Read the model definition and answer for the solid it produces. Units are mm, in the model's axes. Face numbers are marked on the shaded views. A direction names the side the tool comes from. Give positions to 0.01 mm unless a question says otherwise; leave off trailing zeros. Order: outer loops, then holes, each group sorted by start corner. A loop starts at its lowest first (then second) coordinate and runs counter-clockwise, first axis right, second up. Notation, with made-up numbers: (80.25, 30) - (137.25, 30) arc R30 ccw to (137.25, 69) - close; hole circle Ø3 at (-38, -8.75). An arc over 180 degrees is marked (long way). Write each question's results on one line, items separated by ' | '.
from build123d import *

# Parameters (mm, degrees)
F1_DEPTH = 2
F2_DEPTH = 8
F3_DEPTH = 7.25


with BuildPart() as f1:
    # F0 (on Top) → F1 (new body)
    with BuildSketch(Plane.XY):
        with BuildLine():
            Line((4.85, 7.2), (-4.85, 7.2))
            ThreePointArc((-4.85, 7.2), (-6.511701, 6.511701), (-7.2, 4.85))
            Line((-7.2, 4.85), (-7.2, -4.85))
            ThreePointArc((-7.2, -4.85), (-6.511701, -6.511701), (-4.85, -7.2))
            Line((-4.85, -7.2), (4.85, -7.2))
            ThreePointArc((4.85, -7.2), (6.511701, -6.511701), (7.2, -4.85))
            Line((7.2, -4.85), (7.2, 4.85))
            ThreePointArc((7.2, 4.85), (6.511701, 6.511701), (4.85, 7.2))
        make_face()
        with BuildLine():
            ThreePointArc((6.45, -4.85), (5.981371, -5.981371), (4.85, -6.45))
            Line((4.85, -6.45), (-4.85, -6.45))
            ThreePointArc((-4.85, -6.45), (-5.981371, -5.981371), (-6.45, -4.85))
            Line((-6.45, -4.85), (-6.45, 4.85))
            ThreePointArc((-6.45, 4.85), (-5.981371, 5.981371), (-4.85, 6.45))
            Line((-4.85, 6.45), (4.85, 6.45))
            ThreePointArc((4.85, 6.45), (5.981371, 5.981371), (6.45, 4.85))
            Line((6.45, 4.85), (6.45, -4.85))
        make_face(mode=Mode.SUBTRACT)
    extrude(amount=F1_DEPTH)

    # F0 (on Top) → F2 (join)
    with BuildSketch(Plane.XY):
        with BuildLine():
            Line((-4.85, -6.45), (4.85, -6.45))
            ThreePointArc((4.85, -6.45), (5.981371, -5.981371), (6.45, -4.85))
            Line((6.45, -4.85), (6.45, 4.85))
            ThreePointArc((6.45, 4.85), (5.981371, 5.981371), (4.85, 6.45))
            Line((4.85, 6.45), (-4.85, 6.45))
            ThreePointArc((-4.85, 6.45), (-5.981371, 5.981371), (-6.45, 4.85))
            Line((-6.45, 4.85), (-6.45, -4.85))
            ThreePointArc((-6.45, -4.85), (-5.981371, -5.981371), (-4.85, -6.45))
        make_face()
        Polygon((-0.317964, -2.627391), (2.345287, -2.627391), (2.345287, -3.535861), (-2.345287, -3.535861), (0.27015, -0.40403), (0.497567, -0.118938), (0.692111, 0.148224), (0.853782, 0.397456), (0.982582, 0.628757), (1.0809, 0.846013), (1.151127, 1.053108), (1.193263, 1.250043), (1.207309, 1.436817), (1.20249, 1.563637), (1.188034, 1.683508), (1.16394, 1.796432), (1.130208, 1.902408), (1.086839, 2.001435), (1.033833, 2.093515), (0.971189, 2.178647), (0.898907, 2.256831), (0.818258, 2.326871), (0.730511, 2.387573), (0.635667, 2.438935), (0.533726, 2.48096), (0.424687, 2.513645), (0.308551, 2.536992), (0.185317, 2.551), (0.054986, 2.555669), (-0.061934, 2.551), (-0.173625, 2.536992), (-0.280087, 2.513645), (-0.381318, 2.48096), (-0.47732, 2.438935), (-0.568093, 2.387573), (-0.653635, 2.326871), (-0.733948, 2.256831), (-0.807388, 2.17917), (-0.87231, 2.095607), (-0.928716, 2.006142), (-0.976605, 1.910775), (-1.015977, 1.809506), (-1.046832, 1.702335), (-1.069171, 1.589262), (-1.082992, 1.470287), (-2.177937, 1.470287), (-2.168075, 1.699832), (-2.13849, 1.917499), (-2.089182, 2.123287), (-2.02015, 2.317196), (-1.931395, 2.499226), (-1.822917, 2.669378), (-1.694715, 2.82765), (-1.54679, 2.974044), (-1.382204, 3.10572), (-1.204022, 3.219839), (-1.012242, 3.316401), (-0.806865, 3.395406), (-0.587891, 3.456855), (-0.355319, 3.500747), (-0.109151, 3.527082), (0.150615, 3.535861), (0.397344, 3.527717), (0.630699, 3.503287), (0.850682, 3.46257), (1.057292, 3.405567), (1.250528, 3.332277), (1.430392, 3.2427), (1.596882, 3.136836), (1.75, 3.014686), (1.887279, 2.87849), (2.006254, 2.73049), (2.106926, 2.570686), (2.189293, 2.399078), (2.253357, 2.215666), (2.299116, 2.020449), (2.326572, 1.813429), (2.335724, 1.594604), (2.330457, 1.434239), (2.314656, 1.273502), (2.288321, 1.11239), (2.251452, 0.950905), (2.204048, 0.789046), (2.146111, 0.626814), (2.077639, 0.464209), (1.998634, 0.30123), (1.902595, 0.128837), (1.783022, -0.062009), (1.639915, -0.271308), (1.473275, -0.499061), (1.069395, -1.009926), (0.57138, -1.594604), align=None, mode=Mode.SUBTRACT)
    extrude(amount=F2_DEPTH)

    # F0 (on Top) → F3 (join)
    with BuildSketch(Plane.XY):
        Polygon((2.345287, -3.535861), (2.345287, -2.627391), (-0.317964, -2.627391), (0.57138, -1.594604), (1.069395, -1.009926), (1.473275, -0.499061), (1.639915, -0.271308), (1.783022, -0.062009), (1.902595, 0.128837), (1.998634, 0.30123), (2.077639, 0.464209), (2.146111, 0.626814), (2.204048, 0.789046), (2.251452, 0.950905), (2.288321, 1.11239), (2.314656, 1.273502), (2.330457, 1.434239), (2.335724, 1.594604), (2.326572, 1.813429), (2.299116, 2.020449), (2.253357, 2.215666), (2.189293, 2.399078), (2.106926, 2.570686), (2.006254, 2.73049), (1.887279, 2.87849), (1.75, 3.014686), (1.596882, 3.136836), (1.430392, 3.2427), (1.250528, 3.332277), (1.057292, 3.405567), (0.850682, 3.46257), (0.630699, 3.503287), (0.397344, 3.527717), (0.150615, 3.535861), (-0.109151, 3.527082), (-0.355319, 3.500747), (-0.587891, 3.456855), (-0.806865, 3.395406), (-1.012242, 3.316401), (-1.204022, 3.219839), (-1.382204, 3.10572), (-1.54679, 2.974044), (-1.694715, 2.82765), (-1.822917, 2.669378), (-1.931395, 2.499226), (-2.02015, 2.317196), (-2.089182, 2.123287), (-2.13849, 1.917499), (-2.168075, 1.699832), (-2.177937, 1.470287), (-1.082992, 1.470287), (-1.069171, 1.589262), (-1.046832, 1.702335), (-1.015977, 1.809506), (-0.976605, 1.910775), (-0.928716, 2.006142), (-0.87231, 2.095607), (-0.807388, 2.17917), (-0.733948, 2.256831), (-0.653635, 2.326871), (-0.568093, 2.387573), (-0.47732, 2.438935), (-0.381318, 2.48096), (-0.280087, 2.513645), (-0.173625, 2.536992), (-0.061934, 2.551), (0.054986, 2.555669), (0.185317, 2.551), (0.308551, 2.536992), (0.424687, 2.513645), (0.533726, 2.48096), (0.635667, 2.438935), (0.730511, 2.387573), (0.818258, 2.326871), (0.898907, 2.256831), (0.971189, 2.178647), (1.033833, 2.093515), (1.086839, 2.001435), (1.130208, 1.902408), (1.16394, 1.796432), (1.188034, 1.683508), (1.20249, 1.563637), (1.207309, 1.436817), (1.193263, 1.250043), (1.151127, 1.053108), (1.0809, 0.846013), (0.982582, 0.628757), (0.853782, 0.397456), (0.692111, 0.148224), (0.497567, -0.118938), (0.27015, -0.40403), (-2.345287, -3.535861), align=None)
    extrude(amount=F3_DEPTH)


solid = f1.part
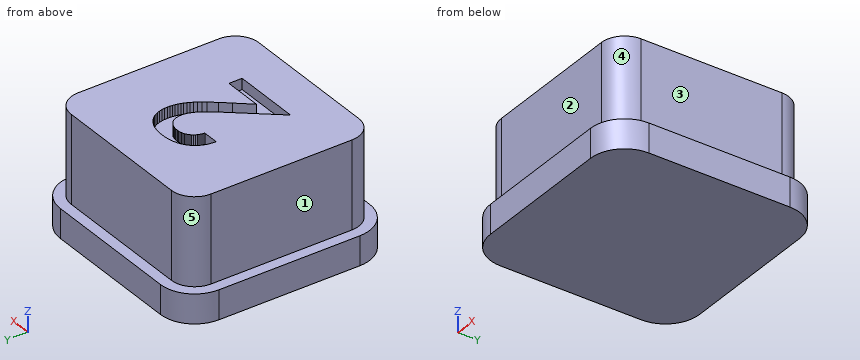
(1) Each of these flat-tipped pins is pushed along its axis until it touches: pin 1 (1.8 mm diameter, centred on y = 2, z = 4.5, fed in from +X); pin 2 (1.8 mm diameter, centred on y = -1, z = 4, fed in from -X); pin 3 (1.8 mm diameter, centred on x = -1.5, z = 4, fed in from -Y). Where does it stop, or does it pass through?
Conclusion:
pin 1: x = 6.45 | pin 2: x = -6.45 | pin 3: y = -6.45
(2) Section C-C (y = -3.25) is taken. Give the vertices of the cut face in (x, z).
Conclusion:
outline: (-7.2, 0) - (7.2, 0) - (7.2, 2) - (6.45, 2) - (6.45, 8) - (2.35, 8) - (2.35, 7.25) - (-2.11, 7.25) - (-2.11, 8) - (-6.45, 8) - (-6.45, 2) - (-7.2, 2) - close
(3) Section A-A (y = 3.75) is taken. Give the vertices of the cut face in (x, z), plus the area to 3 significant figures.
Conclusion:
outline: (-7.2, 0) - (7.2, 0) - (7.2, 2) - (6.45, 2) - (6.45, 8) - (-6.45, 8) - (-6.45, 2) - (-7.2, 2) - close | area: 106 mm^2
(4) Consider probe 1 along Y at (x, z) = (1.5, 7.5); probe 2 along Y at (x, z) = (4.75, 5.5); probe 3 along Z at (x, y) = (6.75, -5). Determine where each line is inside the solid, lowest interval first. Write a range as [from, to].
Conclusion:
probe 1: [-6.45, -3.54], [-2.63, -0.46], [3.2, 6.45] | probe 2: [-6.45, 6.45] | probe 3: [0, 2]
(5) Section B-B (z = 6.75) is taken. Give the vertices of the cut face in (x, y).
Conclusion:
outline: (-6.45, -4.85) arc R1.6 ccw to (-4.85, -6.45) - (4.85, -6.45) arc R1.6 ccw to (6.45, -4.85) - (6.45, 4.85) arc R1.6 ccw to (4.85, 6.45) - (-4.85, 6.45) arc R1.6 ccw to (-6.45, 4.85) - close
(6) For the marked faces 1, 2, 3, 4 and 5, determine the directions among +Z, -Z, +X, -X, +Y, -Y from which every point of the face is accessible in a straight line to the end or side of a thin tool.
Conclusion:
face 1: +Z, -X, +Y, -Y | face 2: +Z, +X, -X, -Y | face 3: +Z, +X, +Y, -Y | face 4: +Z, +X, -Y | face 5: +Z, -X, +Y
